The model under review builds one solid part; all positions refer to its coordinate system, in mm. Coordinates: 2 decimals unless noted, no trailing zeros. Loops run counter-clockwise (first coordinate to the right, second up) from the corner with the lowest first, then second, coordinate; pieces in that order, holes last. Notation, with made-up numbers: M -8.5,61.5 L 49.5,61.5 A24 ccw 49.5,75.5 Z; hole C -16,-19 d2. An arc over 180 degrees is marked long. Write item = value, one per line. Start each with the question number.
Q1. We need section B-B on y = 5.5. Give the boundary of the cut face in (x, z), and give its area (3 significant figures).
Q2. Clearance check with a flat-ended pin moving along its axis: pin 1 Ø2.5 at (x, y) = (5, 5) entering from +Z. State where the tip first meets the part, or that it passes through.
Q3. We need section D-D on y = 1. Give the boundary of the cut face in (x, z), and give its area (3 significant figures).
Q4. We need section C-C on y = 8.5. Give the boundary of the cut face in (x, z).
Q5. We need section A-A on z = 1.05. Count the separate pieces of the cut face and the enclosed holes in it, and give its area (3 significant figures).
Q6. Wall thickness on probe 1 along Y at (x, z) = (5, 1); probe 2 along X at (y, z) = (2.75, 0.5); probe 3 along X at (y, z) = (3, 0.2): over which ranges is each line inside the solid? List them lowest first.
Autodesk Inventor part; units mm, degrees
ref_plane "YZ Plane" through (0, 0, 0) normal (1, 0, 0) x (0, 1, 0)
ref_plane "XZ Plane" through (0, 0, 0) normal (0, 1, 0) x (-1, 0, 0)
ref_plane "XY Plane" through (0, 0, 0) normal (0, 0, 1) x (1, 0, 0)
sketch "Sketch1" plane through (0, 0, 0) normal (0, 0, 1) x (1, 0, 0)
  line L0 (0, 0) -> (60, 0)
  line L1 (60, 0) -> (60, 10)
  line L2 (60, 10) -> (0, 10)
  line L3 (0, 10) -> (0, 0)
  dimension "d0" = 60
  dimension "d1" = 10
extrude "Extrusion1" add sketch "Sketch1" along normal blind 2
fillet "Fillet1" radius 5 4 edges at (60, 10, 1) (60, 0, 1) (0, 0, 1) (0, 10, 1)
sketch "Sketch2" plane through (0, 0, 2) normal (0, 0, 1) x (1, 0, 0)
  arc A0 (5, 10) -> (5, 0) centre (5, 5) ccw
  circle A1 centre (5, 5) radius 1.5
  arc A2 (55, 0) -> (55, 10) centre (55, 5) ccw
  circle A3 centre (55, 5) radius 1.5
  point P0 (0, 0)
  dimension "d5" = 3
  dimension "d6" = 3
extrude "Extrusion2" cut sketch "Sketch2" against normal blind 2
properties part number "Side support 1"
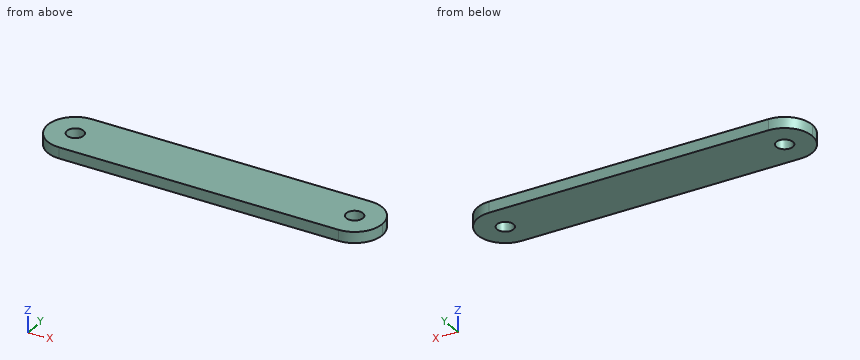
Returned:
q1.outline = M 0.03,0 L 3.59,0 L 3.59,2 L 0.03,2 Z; M 6.41,0 L 53.59,0 L 53.59,2 L 6.41,2 Z; M 56.41,0 L 59.97,0 L 59.97,2 L 56.41,2 Z
q1.area = 109 mm^2
q2.pin_1 = through
q3.outline = M 2,0 L 58,0 L 58,2 L 2,2 Z
q3.area = 112 mm^2
q4.outline = M 1.43,0 L 58.57,0 L 58.57,2 L 1.43,2 Z
q5.separate_pieces = 1
q5.enclosed_holes = 2
q5.area = 564 mm^2
q6.probe_1 = 0 to 3.5, 6.5 to 10
q6.probe_2 = 0.53 to 59.47
q6.probe_3 = 0.42 to 59.58
